from build123d import *

# Parameters (mm, degrees)
F1_DEPTH = 16.764
F2_W     = 70
F2_H     = 90
F3_DEPTH = 4.318
F4_DEPTH = 34.29
F5_W     = 70.352048
F5_H     = 11.088093
F6_DEPTH = 45.974


with BuildPart() as f1:
    # F0 (on Front) → F1 (new body)
    with BuildSketch(Plane.XZ):
        Polygon((35, 39.003629), (35, 45), (-35, 45), (-35, 39.003629), (-28.564712, 39.003629), (28.564712, 39.003629), align=None)
        Polygon((35, -45), (35, 39.003629), (28.564712, 39.003629), (28.564712, -39.003629), (-28.564712, -39.003629), (-28.564712, 39.003629), (-35, 39.003629), (-35, -45), align=None)
    extrude(amount=F1_DEPTH)

    # F2 (on Front) → F3 (join)
    with BuildSketch(Plane.XZ):
        Rectangle(F2_W, F2_H)
    extrude(amount=F3_DEPTH)

    # F0 (on Front) → F4 (join)
    with BuildSketch(Plane.XZ):
        Polygon((35, 39.003629), (35, 45), (-35, 45), (-35, 39.003629), (-28.564712, 39.003629), (28.564712, 39.003629), align=None)
    extrude(amount=-F4_DEPTH)

    # F5 (on Top) → F6 (join)
    with BuildSketch(Plane.XY):
        with Locations((-0.095587, 28.198169)):
            Rectangle(F5_W, F5_H)
    extrude(amount=F6_DEPTH)


solid = f1.part
Build history of the part. All positions in model axes, mm. A direction names the side the tool comes from. Round coordinates to 2 decimals unless told otherwise and drop trailing zeros. Loops run counter-clockwise (first coordinate to the right, second up) from the corner with the lowest first, then second, coordinate; pieces in that order, holes last. Notation, with made-up numbers: (-39, 40) -> (-21, 40) arc R7 cw to (-21, 52) -> close; hole circle Ø7 at (-5, 10). An arc over 180 degrees is marked (long way). Answer in a Markdown table with one row per item.
Item 1: Saw through at D-D (x = 26). Write the cut outline in (y, z).
Answers below:
| item | result |
|---|---|
| outline | (-16.76, -45) -> (0, -45) -> (0, 39) -> (22.65, 39) -> (22.65, 0) -> (33.74, 0) -> (33.74, 39) -> (34.29, 39) -> (34.29, 45) -> (33.74, 45) -> (33.74, 45.97) -> (22.65, 45.97) -> (22.65, 45) -> (-16.76, 45) -> (-16.76, 39) -> (-4.32, 39) -> (-4.32, -39) -> (-16.76, -39) -> close |
Item 2: Saw through at C-C (z = -2). Write the cut outline in (x, y).
Answers below:
| item | result |
|---|---|
| outline | (-35, -16.76) -> (-28.56, -16.76) -> (-28.56, -4.32) -> (28.56, -4.32) -> (28.56, -16.76) -> (35, -16.76) -> (35, 0) -> (-35, 0) -> close |
Item 3: Pin check, flat tips, straight feed: pin 1 (10 mm diameter, centred on y = -2, z = 29.5, fed in from -X); pin 2 (1.5 mm diameter, centred on x = -23, y = 9, fed in from -Z); pin 3 (12 mm diameter, centred on x = -11.5, y = 30, fed in from -Z). Stop position of each tip, or through.
Answers below:
| item | result |
|---|---|
| pin 1 | stops at x = -35 |
| pin 2 | stops at z = 39 |
| pin 3 | stops at z = 0 |
Item 4: Which spindle directions (+Z, -Z, +X, -X, +Y, -Y) get a long thin tool onto all of the face, cutting with end or side? Do faces 5 (the flat face through (-35, -6, 1)), 6 (the flat face through (0, -10, 39.004)), 7 (the flat face through (0, 0, -2)), 8 (the flat face through (35, -6, -1)). Say none if no direction does.
Answers below:
| item | result |
|---|---|
| face 5 | +Z, -Z, -X, -Y |
| face 6 | -Y |
| face 7 | -Z, +X, -X |
| face 8 | +Z, -Z, +X, -Y |
Item 5: Saw through at B-B (y = -11). Write the cut outline in (x, z), and give its area (3 significant figures).
Answers below:
| item | result |
|---|---|
| outline | (-35, -45) -> (35, -45) -> (35, 45) -> (-35, 45) -> close; hole (-28.56, -39) -> (28.56, -39) -> (28.56, 39) -> (-28.56, 39) -> close |
| area | 1,840 mm² |
Item 6: Drill centre lines: L1, parallel to Y at x = -29.5, z = 3.5; L2, parallel to Y at x = 0, z = 1; L3, parallel to X at y = -7.5, z = 16.5. Where is each one in solid material? Low to high. Write a range as [from, to].
Answers below:
| item | result |
|---|---|
| L1 | y = [-16.76, 0], [22.65, 33.74] |
| L2 | y = [-4.32, 0], [22.65, 33.74] |
| L3 | x = [-35, -28.56], [28.56, 35] |
Item 7: Saw through at A-A (z = 17.5). Write the cut outline in (x, y).
Answers below:
| item | result |
|---|---|
| outline | (-35.27, 22.65) -> (35.08, 22.65) -> (35.08, 33.74) -> (-35.27, 33.74) -> close; (-35, -16.76) -> (-28.56, -16.76) -> (-28.56, -4.32) -> (28.56, -4.32) -> (28.56, -16.76) -> (35, -16.76) -> (35, 0) -> (-35, 0) -> close |
Item 8: Mould opens along Z. For faces 1 (the flat face through (0, -10, -39.004)), 2 (the flat face through (0, 3, 45)), 3 (the flat face through (-1, 28, 0)), 4 (the flat face through (0, -4.318, 1)) say: +Z half, -Z half, draft (parallel to the pull), parting line (faces both ways), or undercut.
Answers below:
| item | result |
|---|---|
| face 1 | undercut |
| face 2 | +Z half |
| face 3 | -Z half |
| face 4 | undercut |
